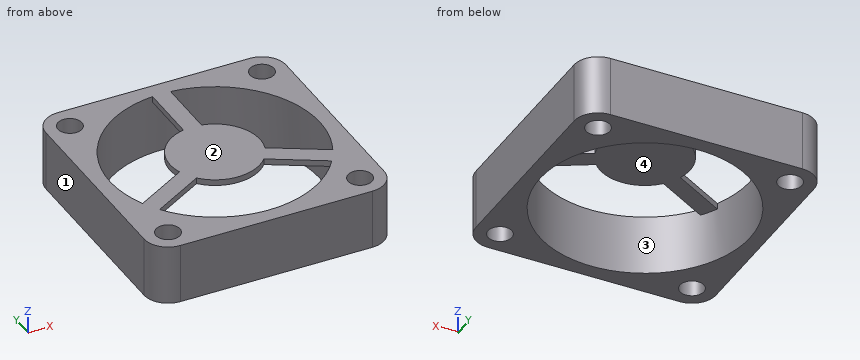
from build123d import *

# Parameters (mm, degrees)
SKETCH_1_R      = 17.5
SKETCH_1_R_2    = 2
EXTRUDE_1_DEPTH = 10
EXTRUDE_START   = -1
EXTRUDE_2_DEPTH = 1


with BuildPart() as part:
    # 草图1 → 凸台-拉伸1 (new body)
    with BuildSketch(Plane.XY):
        with BuildLine():
            Line((-16, -20), (16, -20))
            ThreePointArc((16, -20), (18.828427125, -18.828427125), (20, -16))
            Line((20, -16), (20, 16))
            ThreePointArc((20, 16), (18.828427125, 18.828427125), (16, 20))
            Line((16, 20), (-16, 20))
            ThreePointArc((-16, 20), (-18.828427125, 18.828427125), (-20, 16))
            Line((-20, 16), (-20, -16))
            ThreePointArc((-20, -16), (-18.828427125, -18.828427125), (-16, -20))
        make_face()
        Circle(SKETCH_1_R, mode=Mode.SUBTRACT)
        with Locations((-16, 16)):
            Circle(SKETCH_1_R_2, mode=Mode.SUBTRACT)
        with Locations((16, 16)):
            Circle(SKETCH_1_R_2, mode=Mode.SUBTRACT)
        with Locations((16, -16)):
            Circle(SKETCH_1_R_2, mode=Mode.SUBTRACT)
        with Locations((-16, -16)):
            Circle(SKETCH_1_R_2, mode=Mode.SUBTRACT)
    extrude(amount=EXTRUDE_1_DEPTH)

    # 草图2 → 凸台-拉伸2 (add)
    with BuildSketch(Plane.XY.offset(10).offset(EXTRUDE_START)):
        with BuildLine():
            Line((-1.5, 17.435595774), (-1.5, 7.348469228))
            ThreePointArc((-1.5, 7.348469228), (-6.495190528, 3.75), (-7.113961031, -2.375196508))
            Line((-7.113961031, -2.375196508), (-15.849668871, -7.418759781))
            ThreePointArc((-15.849668871, -7.418759781), (-15.155444566, -8.75), (-14.349668871, -10.016835993))
            Line((-14.349668871, -10.016835993), (-5.613961031, -4.97327272))
            ThreePointArc((-5.613961031, -4.97327272), (0, -7.5), (5.613961031, -4.97327272))
            Line((5.613961031, -4.97327272), (14.349668871, -10.016835993))
            ThreePointArc((14.349668871, -10.016835993), (15.155444566, -8.75), (15.849668871, -7.418759781))
            Line((15.849668871, -7.418759781), (7.113961031, -2.375196508))
            ThreePointArc((7.113961031, -2.375196508), (6.495190528, 3.75), (1.5, 7.348469228))
            Line((1.5, 7.348469228), (1.5, 17.435595774))
            ThreePointArc((1.5, 17.435595774), (0, 17.5), (-1.5, 17.435595774))
        make_face()
    extrude(amount=EXTRUDE_2_DEPTH)


solid = part.part
Model file for the job. Use its own axes, mm. Face numbers are marked on the shaded views. Give positions to 0.01 mm unless a question says otherwise; leave off trailing zeros. Loops run counter-clockwise (first coordinate to the right, second up) from the corner with the lowest first, then second, coordinate; pieces in that order, holes last. Notation, with made-up numbers: (30.25, -8.5) -> (43.25, -8.5) arc R9 ccw to (43.25, -1.5) -> close; hole circle Ø5 at (-27, -9.75). An arc over 180 degrees is marked (long way). Use a Markdown table: item, result. Add a question column.
(1) Slice it at D-D on x = -8. List the corners of the cut face in (y, z).
(2) Slice it at B-B on z = 4. List the corners of the cut face in (x, y), and give its area (3 significant figures).
(3) Slice it at C-C on y = 15.5. List the corners of the cut face in (x, z).
(4) Wall check: line 1 along Y through (x, z) = (-16, 2.25); line 2 along Y through (x, z) = (0, 5.25). Give the ranges that are in metal, low to high.
(5) Slice it at A-A on x = 0. List the corners of the cut face in (y, z).
(6) Mould opens along X. For the marked faces 1, 2, 3 and 4 say: +X half, -X half, draft (parallel to the pull), parting line (faces both ways), or undercut.
(7) Drop a flat-ended pin along its axis: pin 1 Ø14 at (x, y) = (-2, 5) entering from -Z. Give the stop position or say it passes through.
Filled sheet:
| question | item | result |
|---|---|---|
| 1 | outline | (-20, 0) -> (-15.56, 0) -> (-15.56, 10) -> (-20, 10) -> close; (-6.35, 9) -> (-2.89, 9) -> (-2.89, 10) -> (-6.35, 10) -> close; (15.56, 0) -> (20, 0) -> (20, 10) -> (15.56, 10) -> close |
| 2 | outline | (-20, -16) arc R4 ccw to (-16, -20) -> (16, -20) arc R4 ccw to (20, -16) -> (20, 16) arc R4 ccw to (16, 20) -> (-16, 20) arc R4 ccw to (-20, 16) -> close; hole circle Ø4 at (-16, -16); hole circle Ø4 at (-16, 16); hole circle Ø35 at (0, 0); hole circle Ø4 at (16, -16); hole circle Ø4 at (16, 16) |
| 2 | area | 574 mm2 |
| 3 | outline | (-20, 0) -> (-17.94, 0) -> (-17.94, 10) -> (-20, 10) -> close; (-14.06, 0) -> (-8.12, 0) -> (-8.12, 10) -> (-14.06, 10) -> close; (-1.5, 9) -> (1.5, 9) -> (1.5, 10) -> (-1.5, 10) -> close; (8.12, 0) -> (14.06, 0) -> (14.06, 10) -> (8.12, 10) -> close; (17.94, 0) -> (20, 0) -> (20, 10) -> (17.94, 10) -> close |
| 4 | line 1 | -20 to -18, -14 to -7.09, 7.09 to 14, 18 to 20 |
| 4 | line 2 | -20 to -17.5, 17.5 to 20 |
| 5 | outline | (-20, 0) -> (-17.5, 0) -> (-17.5, 10) -> (-20, 10) -> close; (-7.5, 9) -> (17.5, 9) -> (17.5, 0) -> (20, 0) -> (20, 10) -> (-7.5, 10) -> close |
| 6 | face 1 | -X half |
| 6 | face 2 | draft |
| 6 | face 3 | undercut |
| 6 | face 4 | undercut |
| 7 | pin 1 | z = 9 |
